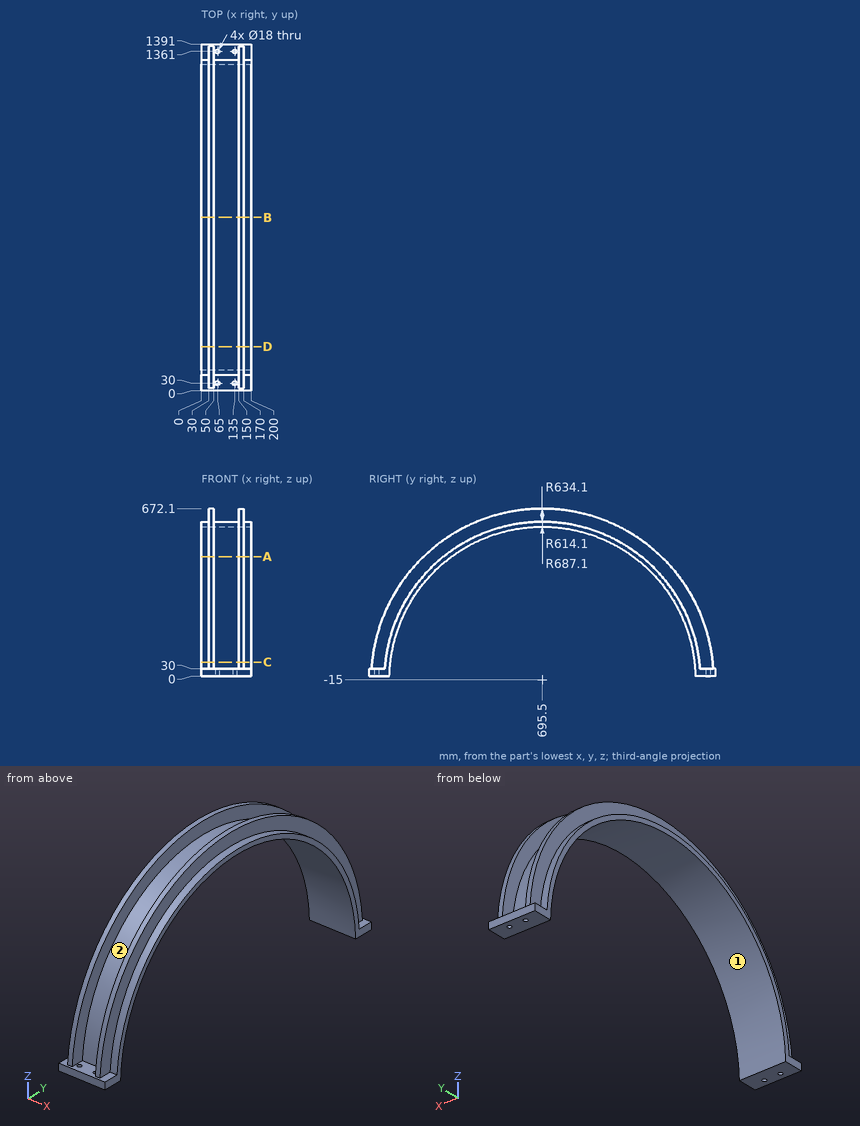
Answer from the drawing. Dimensions are ordinates in mm from the lowest x, y and z of the part. Round coordinates to 2 decimals unless told otherwise and drop trailing zeros. Write each loop counter-clockwise with the first axis right and the second up, starting at its lowest first coordinate (ties: lowest second). Pieces come first, ordered by that corner, then holes.
1. The part is cut by section B-B, the plane y = 695.5. Determine the outline of the cut face in (x, z), then the cut area to 3 significant figures.
2. Determine the mould class of the marked faces 1 and 2 for opening direction X: pulls with the +X half, pulls with the -X half, needs draft (parallel to the pull), parting line crosses it, or undercut.
3. Straight lines are drawn through the part: L1, parallel to X at y = 1361, z = 21; L2, parallel to Y at x = 135, z = 9.5; L3, parallel to Y at x = 135, z = 24. For each, find the intervals that lie inside material, in ascending order.
4. The part is cut by section A-A, the plane z = 479.5. Determine the outline of the cut face in (x, y), then the cut area to 3 significant figures.
5. Given pin 1 Ø6 at (x, z) = (101, 284.5) entering from -Y; pin 2 Ø4 at (x, y) = (63.5, 374) entering from -Z; pin 3 Ø1.5 at (x, z) = (115, 233) entering from -Y, each flat-ended and moving along its own axis, determine where each tip first touches the part or whether it passes through.
6. The part is cut by section C-C, the plane z = 56. Determine the outline of the cut face in (x, y), then the cut area to 3 significant figures.
7. The part is cut by section D-D, the plane y = 176. Determine the outline of the cut face in (x, z), then the cut area to 3 significant figures.
Values:
1. outline: (0, 599.1) - (200, 599.1) - (200, 619.1) - (170, 619.1) - (170, 672.1) - (150, 672.1) - (150, 619.1) - (50, 619.1) - (50, 672.1) - (30, 672.1) - (30, 619.1) - (0, 619.1) - close
1. area: 6,120 mm2
2. face 1: needs draft
2. face 2: undercut
3. L1: x = 0 to 56, 74 to 126, 144 to 200
3. L2: y = 0 to 21, 39 to 81.89, 1309.11 to 1352, 1370 to 1391
3. L3: y = 0 to 21, 39 to 82.64, 1308.36 to 1352, 1370 to 1391
4. outline: (0, 298.57) - (30, 298.57) - (30, 218.45) - (50, 218.45) - (50, 298.57) - (150, 298.57) - (150, 218.45) - (170, 218.45) - (170, 298.57) - (200, 298.57) - (200, 331.37) - (0, 331.37) - close; (0, 1059.63) - (200, 1059.63) - (200, 1092.43) - (170, 1092.43) - (170, 1172.55) - (150, 1172.55) - (150, 1092.43) - (50, 1092.43) - (50, 1172.55) - (30, 1172.55) - (30, 1092.43) - (0, 1092.43) - close
4. area: 19,500 mm2
5. pin 1: stops at y = 134.99
5. pin 2: stops at z = 506.98
5. pin 3: stops at y = 111.59
6. outline: (0, 65.39) - (30, 65.39) - (30, 12.08) - (50, 12.08) - (50, 65.39) - (150, 65.39) - (150, 12.08) - (170, 12.08) - (170, 65.39) - (200, 65.39) - (200, 85.52) - (0, 85.52) - close; (0, 1305.48) - (200, 1305.48) - (200, 1325.61) - (170, 1325.61) - (170, 1378.92) - (150, 1378.92) - (150, 1325.61) - (50, 1325.61) - (50, 1378.92) - (30, 1378.92) - (30, 1325.61) - (0, 1325.61) - close
6. area: 12,300 mm2
7. outline: (0, 312.47) - (200, 312.47) - (200, 348.6) - (170, 348.6) - (170, 434.7) - (150, 434.7) - (150, 348.6) - (50, 348.6) - (50, 434.7) - (30, 434.7) - (30, 348.6) - (0, 348.6) - close
7. area: 10,700 mm2
